```python
from build123d import *

# Parameters (mm, degrees)
ESQUISSE1_R             = 50
BOSS_EXTRU_1_DEPTH      = 17
COQUE1_T                = -2
ESQUISSE2_R             = 4.5
ENL_V_MAT_EXTRU_3_DEPTH = 73.725511342
CHANFREIN1_SIZE         = 1
ESQUISSE3_R             = 50
ESQUISSE3_R_2           = 44.5
BOSS_EXTRU_2_DEPTH      = 1
ESQUISSE4_R             = 45.5
ESQUISSE4_R_2           = 44.5
BOSS_EXTRU_3_DEPTH      = 10
ESQUISSE5_W             = 4
ESQUISSE5_H             = 2.5
ENL_V_MAT_EXTRU_4_DEPTH = 9


with BuildPart() as part:
    # Esquisse1 → Boss.-Extru.1 (new body)
    with BuildSketch(Plane(origin=(0, 0, 0), x_dir=(1, 0, 0), z_dir=(0, 1, 0))):
        with Locations(Location((0, 0, 0), (0, 0, 270))):
            Circle(ESQUISSE1_R)
    extrude(amount=BOSS_EXTRU_1_DEPTH)

    # Coque1
    coque1_openings = [part.faces().sort_by_distance(p)[0] for p in [
        (0, 17, 0),
    ]]
    offset(amount=COQUE1_T, openings=coque1_openings, kind=Kind.INTERSECTION)

    # Esquisse2 → Enlèv. mat.-Extru.3 (cut, through all)
    with BuildSketch(Plane(origin=(0, 0, 0), x_dir=(1, 0, 0), z_dir=(0, 1, 0))):
        with Locations(Location((0, 0, 0), (0, 0, 270))):
            Circle(ESQUISSE2_R)
    extrude(amount=ENL_V_MAT_EXTRU_3_DEPTH, mode=Mode.SUBTRACT)

    # Chanfrein1
    chanfrein1_edges = [part.edges().sort_by_distance(p)[0] for p in [
        (0, 0, -4.5),
    ]]
    chamfer(chanfrein1_edges, length=CHANFREIN1_SIZE)

    # Esquisse3 → Boss.-Extru.2 (add)
    with BuildSketch(Plane(origin=(0, 10, 0), x_dir=(1, 0, 0), z_dir=(0, 1, 0))):
        with Locations(Location((0, 0, 0), (0, 0, 270))):
            Circle(ESQUISSE3_R)
        with Locations(Location((0, 0, 0), (0, 0, 270))):
            Circle(ESQUISSE3_R_2, mode=Mode.SUBTRACT)
    extrude(amount=BOSS_EXTRU_2_DEPTH)

    # Esquisse4 → Boss.-Extru.3 (add)
    with BuildSketch(Plane(origin=(0, 10, 0), x_dir=(1, 0, 0), z_dir=(0, 1, 0))):
        with Locations(Location((0, 0, 0), (0, 0, 270))):
            Circle(ESQUISSE4_R)
        with Locations(Location((0, 0, 0), (0, 0, 270))):
            Circle(ESQUISSE4_R_2, mode=Mode.SUBTRACT)
    extrude(amount=BOSS_EXTRU_3_DEPTH)

    # Esquisse5 → Enlèv. mat.-Extru.4 (cut)
    with BuildSketch(Plane(origin=(0, 20, 0), x_dir=(1, 0, 0), z_dir=(0, 1, 0))):
        with Locations((0, 45.25)):
            Rectangle(ESQUISSE5_W, ESQUISSE5_H)
    extrude(amount=-ENL_V_MAT_EXTRU_4_DEPTH, mode=Mode.SUBTRACT)


solid = part.part
```
Geometry check sheet. Reference: the model listing, model coordinates, mm. A direction names the side the tool comes from. Coordinates: 2 decimals unless noted, no trailing zeros. Order: outer loops, then holes, each group sorted by start corner. A loop starts at its lowest first (then second) coordinate and runs counter-clockwise, first axis right, second up.
Q1. Tool access check on faces 4 (the face through (44, 20, 10)), 5 (the face through (19, 17, -45)), 6 (the face through (-42.4, 10, 14)). Record the directions out of +Z, -Z, +X, -X, +Y, -Y that give a thin tool (end or side, any length) a straight path to the whole face; none if there is none.
Reply:
face 4: +Z, -Z, +X, -X, +Y
face 5: +Y
face 6: none
Q2. Sectioned sample at A-A on y = 13. Record the cut outline in (x, z).
Reply:
outline: circle Ø100 at (0, 0); (-2, -45.46) - (-2, -44.46) arc R44.5 cw (long way) to (2, -44.46) - (2, -45.46) arc R45.5 ccw (long way) to start; hole circle Ø96 at (0, 0)
Q3. Draft check along X on faces 1 (the face through (-10, 0, -1)), 2 (the face through (13.367, 14.93, 42.445)), 3 (the face through (15.02, 8.38, 47.69)). Enter one of: released by +X, released by -X, zero draft, split by the parting line, or undercut.
Reply:
face 1: zero draft
face 2: undercut
face 3: split by the parting line
Q4. Depth check by flat-ended pin: pin 1 Ø8 at (y, z) = (17.5, 18) entering from -X; pin 2 Ø1 at (y, z) = (4, 7.5) entering from -X; pin 3 Ø6 at (x, y) = (13, 16.5) entering from +Z. Enter the tip coordinate at first touch or a pass-through.
Reply:
pin 1: stops at x = -47.99
pin 2: stops at x = -49.51
pin 3: stops at z = 48.99
Q5. Sectioned sample at B-B on z = 0. Record the cut outline in (x, y), and give its area (3 significant figures).
Reply:
outline: (-50, 0) - (-5.5, 0) - (-4.5, 1) - (-4.5, 2) - (-48, 2) - (-48, 10) - (-44.5, 10) - (-44.5, 20) - (-45.5, 20) - (-45.5, 11) - (-48, 11) - (-48, 17) - (-50, 17) - close; (4.5, 1) - (5.5, 0) - (50, 0) - (50, 17) - (48, 17) - (48, 11) - (45.5, 11) - (45.5, 20) - (44.5, 20) - (44.5, 10) - (48, 10) - (48, 2) - (4.5, 2) - close
area: 266 mm2
Q6. Thickness scan on probe 1 along X at (y, z) = (12.25, 0); probe 2 along X at (y, z) = (1.5, 0); probe 3 along X at (y, z) = (4.25, 0). Record the ranges inside material, lowest first.
Reply:
probe 1: x = -50 to -48, -45.5 to -44.5, 44.5 to 45.5, 48 to 50
probe 2: x = -50 to -4.5, 4.5 to 50
probe 3: x = -50 to -48, 48 to 50
Q7. Sectioned sample at C-C on x = 39. Record the cut outline in (y, z), and give its area (3 significant figures).
Reply:
outline: (0, -31.29) - (17, -31.29) - (17, -27.98) - (11, -27.98) - (11, -23.44) - (20, -23.44) - (20, -21.43) - (10, -21.43) - (10, -27.98) - (2, -27.98) - (2, 27.98) - (10, 27.98) - (10, 21.43) - (20, 21.43) - (20, 23.44) - (11, 23.44) - (11, 27.98) - (17, 27.98) - (17, 31.29) - (0, 31.29) - close
area: 274 mm2
Q8. Sectioned sample at D-D on y = 6.5. Record the cut outline in (x, z).
Reply:
outline: circle Ø100 at (0, 0); hole circle Ø96 at (0, 0)
